For this review, take the finished solid that the model builds, in its own axes (mm). A direction names the side the tool comes from. Round coordinates to 2 decimals unless told otherwise and drop trailing zeros. Loops run counter-clockwise (first coordinate to the right, second up) from the corner with the lowest first, then second, coordinate; pieces in that order, holes last.
1) Mouldability with a two-part tool opening along Y and no side actions: class faces 1 (the flat face through (11, 13.1, 13)), 2 (the flat face through (11, 3.653, 12)), 3 (the flat face through (13, 9, 20)) as pulls with the +Y half, pulls with the -Y half, needs draft (parallel to the pull), parting line crosses it, or undercut.
2) Take a section at A-A (x = 5). State the section outline as (y, z) points.
3) Wall thickness on L1, parallel to X at y = 18, z = 4.1; L2, parallel to Z at x = 14.5, y = 17; L3, parallel to Y at x = 18, z = 4.5: over which ranges is each line inside the solid? List them lowest first.
4) Take a section at D-D (y = 11). State the section outline as (x, z) points.
5) Take a section at C-C (z = 10.5). State the section outline as (x, y) points, then the cut area to 3 significant figures.
6) Take a section at B-B (z = 2). State the section outline as (x, y) points (3 decimals), then the cut area to 3 significant figures.
7) Tool access review of faces 4 (the flat face through (2.7, 19.4, 3)), 5 (the flat face through (11, 21.8, 2)): name each direction out of +Z, -Z, +X, -X, +Y, -Y from which nothing blocks a thin tool from reaching the whole face with its end or side.
8) Insertion check: pin 1 (8 mm diameter, centred on y = 19.5, z = 6, fed in from +X); pin 2 (1 mm diameter, centred on x = 19.5, z = 17, fed in from +Y); pin 3 (3.5 mm diameter, centred on x = 18, y = 18, fed in from -Z); pin 4 (1.5 mm diameter, centred on x = 12, z = 9, fed in from +Y). Each pin has a flat end and moves straight along its axis. Give the tip position at first contact, or say it passes through.
```python
from build123d import *

# Parameters (mm, degrees)
SKETCH_W        = 21.8
SKETCH_H        = 21.8
PAD_DEPTH       = 5
PAD001_DEPTH    = 15
SKETCH002_R     = 1.6
POCKET_DEPTH    = 20.001
POCKET001_DEPTH = 3
POCKET002_DEPTH = 15


with BuildPart() as part:
    # Sketch → Pad (new body)
    with BuildSketch(Plane.XY):
        with Locations((10.9, 10.9)):
            Rectangle(SKETCH_W, SKETCH_H)
    extrude(amount=PAD_DEPTH)

    # Sketch001 (on Face6 of Pad) → Pad001 (join)
    with BuildSketch(Plane.XY.offset(5)):
        Polygon((1, 3.652697), (10.9, 20.8), (20.8, 3.652697), align=None)
    extrude(amount=PAD001_DEPTH)

    # Sketch002 (on Face4 of Pad001) → Pocket (cut, through all)
    with BuildSketch(Plane(origin=(0, 0, 0), x_dir=(1, 0, 0), z_dir=(0, 0, -1))):
        with Locations((4, -18)):
            Circle(SKETCH002_R)
        with Locations((18, -18)):
            Circle(SKETCH002_R)
    extrude(amount=-POCKET_DEPTH, mode=Mode.SUBTRACT)

    # Sketch003 (on Face4 of Pocket) → Pocket001 (cut)
    with BuildSketch(Plane(origin=(0, 0, 0), x_dir=(1, 0, 0), z_dir=(0, 0, -1))):
        Polygon((6.775, -19.602147), (6.775, -16.397853), (4, -14.795706), (1.225, -16.397853), (1.225, -19.602147), (4, -21.204294), align=None)
        Polygon((20.775, -19.602147), (20.775, -16.397853), (18, -14.795706), (15.225, -16.397853), (15.225, -19.602147), (18, -21.204294), align=None)
    extrude(amount=-POCKET001_DEPTH, mode=Mode.SUBTRACT)

    # Sketch004 (on Face26 of Pocket001) → Pocket002 (cut)
    with BuildSketch(Plane.XY.offset(20)):
        with BuildLine():
            ThreePointArc((9.467029, 13.1), (11, 8.4), (12.532971, 13.1))
            Line((9.467029, 13.1), (12.532971, 13.1))
        make_face()
    extrude(amount=-POCKET002_DEPTH, mode=Mode.SUBTRACT)


solid = part.part
```
Response:
1. face 1: undercut
1. face 2: pulls with the -Y half
1. face 3: needs draft
2. outline: (0, 0) - (15.37, 0) - (15.37, 3) - (16.75, 3) - (16.75, 5) - (10.58, 5) - (10.58, 20) - (3.65, 20) - (3.65, 5) - (0, 5) - close; (19.25, 3) - (20.63, 3) - (20.63, 0) - (21.8, 0) - (21.8, 5) - (19.25, 5) - close
3. L1: x = 0 to 2.4, 5.6 to 16.4, 19.6 to 21.8
3. L2: z = 0 to 5
3. L3: y = 0 to 16.4, 19.6 to 21.8
4. outline: (0, 0) - (21.8, 0) - (21.8, 5) - (16.56, 5) - (16.56, 20) - (13.6, 20) - (13.6, 5) - (8.4, 5) - (8.4, 20) - (5.24, 20) - (5.24, 5) - (0, 5) - close
5. outline: (1, 3.65) - (20.8, 3.65) - (10.9, 20.8) - close; hole (9.47, 13.1) arc R2.6 ccw (long way) to (12.53, 13.1) - close
5. area: 150 mm2
6. outline: (0, 0) - (21.8, 0) - (21.8, 21.8) - (0, 21.8) - close; hole (1.225, 16.398) - (4, 14.796) - (6.775, 16.398) - (6.775, 19.602) - (4, 21.204) - (1.225, 19.602) - close; hole (15.225, 16.398) - (18, 14.796) - (20.775, 16.398) - (20.775, 19.602) - (18, 21.204) - (15.225, 19.602) - close
6. area: 422 mm2
7. face 4: -Z
7. face 5: +Z, -Z, +X, -X, +Y
8. pin 1: stops at x = 21.8
8. pin 2: stops at y = 6.77
8. pin 3: stops at z = 3
8. pin 4: stops at y = 20.19
